Geometry check sheet. Reference: the model listing, model coordinates, mm. A direction names the side the tool comes from. Give positions to 0.01 mm unless a question says otherwise; leave off trailing zeros. Write each loop counter-clockwise with the first axis right and the second up, starting at its lowest first coordinate (ties: lowest second). Pieces come first, ordered by that corner, then holes.
(1) Thickness scan on line 1 along Z through (x, y) = (3, 2.75); line 2 along Z through (x, y) = (-3.75, 1.25); line 3 along Z through (x, y) = (-6.75, 2.25). Record the ranges inside material, lowest first.
(2) Depth check by flat-ended pin: P1, Ø0.8, axis at y = 2.5, z = -6.5, coming from the -X side; P2, Ø7, axis at x = 6, z = 7.5, coming from the +Y side; P3, Ø1.6, axis at x = 8.5, y = 2.5, coming from the +Z side; P4, Ø1.5, axis at x = -7.5, z = -10, coming from the +Y side. Enter the tip coordinate at first touch or a pass-through.
(3) Mould release check, pull along X, two halves, no side actions. Record for faces 1 (the flat face through (-9.35, 2, 7)), 2 (the flat face through (-9.35, 2, 0)), 3 (the flat face through (0, 1, 11.5)), 4 (the flat face through (-11, 2, 0)): +X half, -X half, draft (parallel to the pull), parting line (faces both ways), or undercut.
(4) Cross-section at C-C (y = 0.75). Record the boundary of the cut face in (x, z).
(5) Cross-section at B-B (z = -5.5). Record the boundary of the cut face in (x, y).
(6) Cross-section at A-A (x = -3.75). Record the boundary of the cut face in (y, z), and give its area (3 significant figures).
(7) Tool access check on faces 5 (the flat face through (-8, 3, 9)), 6 (the flat face through (-11, 3, -12)), 7 (the flat face through (-1.5, 2, 9)), 8 (the flat face through (-10, 2, 4.65)), 9 (the flat face through (10, 2, -1.5)). Record the directions out of +Z, -Z, +X, -X, +Y, -Y that give a thin tool (end or side, any length) a straight path to the whole face; none if there is none.
(8) Cross-section at D-D (x = 3.25). Record the boundary of the cut face in (y, z).
```python
from build123d import *

# Parameters (mm, degrees)
SKETCH1_W               = 25
SKETCH1_H               = 23
BOSS_EXTRUDE1_DEPTH     = 1.5
SKETCH2_W               = 22
SKETCH2_H               = 20
SKETCH2_W_2             = 18.7
SKETCH2_H_2             = 17
BOSS_EXTRUDE2_DEPTH     = 1.5
SKETCH4_W               = 12
SKETCH4_H               = 7.8
CUT_EXTRUDE2_DEPTH      = 2.5
CUT_EXTRUDE2_DEPTH_BACK = 2.5
SKETCH5_W               = 13.5
SKETCH5_H               = 9.3
CUT_EXTRUDE3_DEPTH      = 4
SKETCH6_W               = 1.65
SKETCH6_H               = 3
SKETCH6_W_2             = 3
SKETCH6_H_2             = 1.5
CUT_EXTRUDE4_DEPTH      = 1.5
SKETCH7_W               = 23.5
SKETCH7_H               = 7
BOSS_EXTRUDE3_DEPTH     = 2
SKETCH8_W               = 11.7
SKETCH8_H               = 0.15
CUT_EXTRUDE5_DEPTH      = 5.5


with BuildPart() as part:
    # Sketch1 → Boss-Extrude1 (new body)
    with BuildSketch(Plane(origin=(0, 0, 0), x_dir=(1, 0, 0), z_dir=(0, 1, 0))):
        Rectangle(SKETCH1_W, SKETCH1_H)
    extrude(amount=BOSS_EXTRUDE1_DEPTH)

    # Sketch2 → Boss-Extrude2 (add)
    with BuildSketch(Plane(origin=(0, 1.5, 0), x_dir=(1, 0, 0), z_dir=(0, 1, 0))):
        Rectangle(SKETCH2_W, SKETCH2_H)
        Rectangle(SKETCH2_W_2, SKETCH2_H_2, mode=Mode.SUBTRACT)
    extrude(amount=BOSS_EXTRUDE2_DEPTH)

    # Sketch4 → Cut-Extrude2 (cut, two sides)
    with BuildSketch(Plane(origin=(0, 1.5, 0), x_dir=(1, 0, 0), z_dir=(0, 1, 0))) as cut_extrude2_sk:
        with Locations((-5, 6.1)):
            Rectangle(SKETCH4_W, SKETCH4_H)
    extrude(amount=CUT_EXTRUDE2_DEPTH, mode=Mode.SUBTRACT)
    extrude(cut_extrude2_sk.sketch, amount=-CUT_EXTRUDE2_DEPTH_BACK, mode=Mode.SUBTRACT)

    # Sketch5 → Cut-Extrude3 (cut, through all)
    with BuildSketch(Plane.XZ):
        with Locations((-5.75, -6.85)):
            Rectangle(SKETCH5_W, SKETCH5_H)
    extrude(amount=-CUT_EXTRUDE3_DEPTH, mode=Mode.SUBTRACT)

    # Sketch6 → Cut-Extrude4 (cut)
    with BuildSketch(Plane(origin=(0, 3, 0), x_dir=(1, 0, 0), z_dir=(0, 1, 0))):
        with Locations((-10.175, -3.15)):
            Rectangle(SKETCH6_W, SKETCH6_H)
        with Locations((0, -9.25)):
            Rectangle(SKETCH6_W_2, SKETCH6_H_2)
        with Locations((10.175, 0)):
            Rectangle(SKETCH6_W, SKETCH6_H)
        with Locations((5.175, 9.25)):
            Rectangle(SKETCH6_W_2, SKETCH6_H_2)
    extrude(amount=-CUT_EXTRUDE4_DEPTH, mode=Mode.SUBTRACT)

    # Sketch7 → Boss-Extrude3 (add)
    with BuildSketch(Plane(origin=(0, 0, -11.5), x_dir=(-1, 0, 0), z_dir=(0, 0, -1))):
        with Locations((-0.75, 3.5)):
            Rectangle(SKETCH7_W, SKETCH7_H)
    extrude(amount=BOSS_EXTRUDE3_DEPTH)

    # Sketch8 → Cut-Extrude5 (cut)
    with BuildSketch(Plane(origin=(0, 7, 0), x_dir=(1, 0, 0), z_dir=(0, 1, 0))):
        with Locations((6.65, 11.575)):
            Rectangle(SKETCH8_W, SKETCH8_H)
    extrude(amount=-CUT_EXTRUDE5_DEPTH, mode=Mode.SUBTRACT)


solid = part.part
```
Reply:
1. line 1: z = -13.5 to -11.65, -10 to -8.5, 8.5 to 10
1. line 2: z = -13.5 to -11.5, -2.2 to 11.5
1. line 3: z = -13.5 to -11.5, 8.5 to 10
2. P1: stops at x = 9.35
2. P2: stops at y = 3
2. P3: stops at z = 10
2. P4: passes through
3. face 1: undercut
3. face 2: undercut
3. face 3: draft
3. face 4: -X half
4. outline: (-12.5, -2.2) - (1, -2.2) - (1, -11.5) - (-11, -11.5) - (-11, -13.5) - (12.5, -13.5) - (12.5, 11.5) - (-12.5, 11.5) - close
5. outline: (1, 0) - (12.5, 0) - (12.5, 1.5) - (11, 1.5) - (11, 3) - (9.35, 3) - (9.35, 1.5) - (1, 1.5) - close
6. outline: (0, -13.5) - (7, -13.5) - (7, -11.5) - (0, -11.5) - close; (0, -2.2) - (1.5, -2.2) - (1.5, 8.5) - (3, 8.5) - (3, 10) - (1.5, 10) - (1.5, 11.5) - (0, 11.5) - close
6. area: 36.8 mm2
7. face 5: +Z, +X, -X, +Y
7. face 6: -Z, -X, +Y, -Y
7. face 7: +Z, +Y
7. face 8: -X, +Y
7. face 9: +X, +Y
8. outline: (0, -13.5) - (7, -13.5) - (7, -11.65) - (1.5, -11.65) - (1.5, -10) - (3, -10) - (3, -8.5) - (1.5, -8.5) - (1.5, 8.5) - (3, 8.5) - (3, 10) - (1.5, 10) - (1.5, 11.5) - (0, 11.5) - close
